Here's how the part is built. I have some questions about the finished solid (model axes, mm). Face numbers are marked on the shaded views. A direction names the side the tool comes from. Round coordinates to 2 decimals unless told otherwise and drop trailing zeros. Order: outer loops, then holes, each group sorted by start corner. A loop starts at its lowest first (then second) coordinate and runs counter-clockwise, first axis right, second up. Notation, with made-up numbers: (-9, 4.25) - (4, 4.25) arc R11 cw to (4, 10.25) - close; hole circle Ø1 at (52, -6.75). An arc over 180 degrees is marked (long way). Answer as a JSON object with one key per item and string values.
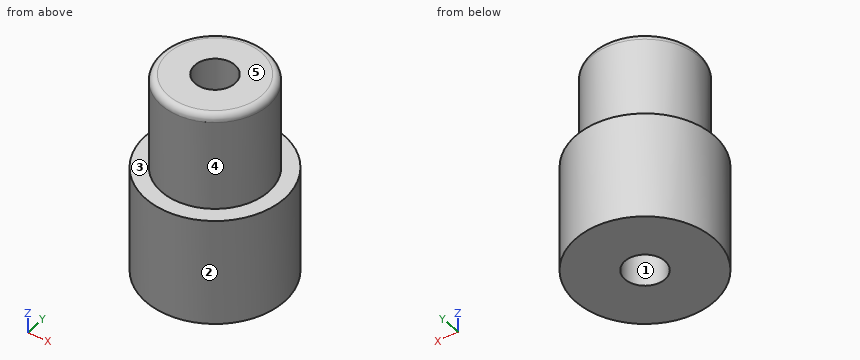
```python
from build123d import *

# Parameters (mm, degrees)
F0_R     = 10
F1_DEPTH = 15.5
F2_R     = 7.75
F3_DEPTH = 14
F4_R     = 2.898353
F5_DEPTH = 31
F6_R     = 1


with BuildPart() as f1:
    # F0 (on Top) → F1 (new body)
    with BuildSketch(Plane.XY):
        Circle(F0_R)
    extrude(amount=F1_DEPTH)

    # F2 (on face) → F3 (join)
    with BuildSketch(Plane.XY.offset(15.5)):
        Circle(F2_R)
    extrude(amount=F3_DEPTH)

    # F4 (on face) → F5 (cut)
    with BuildSketch(Plane.XY.offset(29.5)):
        Circle(F4_R)
    extrude(amount=-F5_DEPTH, mode=Mode.SUBTRACT)

    # F6
    f6_edges = [f1.edges().sort_by_distance(p)[0] for p in [
        (-7.75, 0, 29.5),
    ]]
    fillet(f6_edges, radius=F6_R)


solid = f1.part
```
1. Imagine slicing it at D-D (y = -8.25). List the corners of the cut face in (x, z) for me, plus the area to 3 significant figures.
Responses:
{"outline": "(-5.65, 0) - (5.65, 0) - (5.65, 15.5) - (-5.65, 15.5) - close", "area": "175 mm2"}
2. For P1, Ø10, axis at y = -6, z = 8, coming from the -X side; P2, Ø2, axis at y = 0, z = 21.5, coming from the -X side; P3, Ø8, axis at y = -7, z = 8.5, coming from the +X side, each with a flat end and sliding along its axis, tell me the tip position at first contact or that it passes through.
Responses:
{"P1": "x = -9.95", "P2": "x = -7.75", "P3": "x = 9.54"}
3. Imagine slicing it at C-C (z = 19). List the corners of the cut face in (x, y) for me.
Responses:
{"outline": "circle Ø15.5 at (0, 0); hole circle Ø5.8 at (0, 0)"}
4. Imagine slicing it at A-A (y = 0). List the corners of the cut face in (x, z) for me, plus the area to 3 significant figures.
Responses:
{"outline": "(-10, 0) - (-2.9, 0) - (-2.9, 29.5) - (-6.75, 29.5) arc R1 ccw to (-7.75, 28.5) - (-7.75, 15.5) - (-10, 15.5) - close; (2.9, 0) - (10, 0) - (10, 15.5) - (7.75, 15.5) - (7.75, 28.5) arc R1 ccw to (6.75, 29.5) - (2.9, 29.5) - close", "area": "356 mm2"}
5. If I drill on L1, parallel to Y at x = 0, z = 21; L2, parallel to X at y = 1, z = 1.5; L3, parallel to Y at x = -2, z = 16.75, over which ranges is the centre line in solid material (lowest first)? Write a range as [from, to].
Responses:
{"L1": "[-7.75, -2.9], [2.9, 7.75]", "L2": "[-9.95, -2.72], [2.72, 9.95]", "L3": "[-7.49, -2.1], [2.1, 7.49]"}
6. For the marked faces 4 and 5, which set-ups out of +Z, -Z, +X, -X, +Y, -Y let a thin tool reach every point of the face, with its end or its side?
Responses:
{"face 4": "+Z", "face 5": "+Z, +X, -X, +Y, -Y"}
7. Thinking about a two-plate mould opening in X: for the marked faces 1, 2 and 3, which applies, pulls with the +X half, pulls with the -X half, needs draft (parallel to the pull), parting line crosses it, or undercut?
Responses:
{"face 1": "undercut", "face 2": "parting line crosses it", "face 3": "needs draft"}
